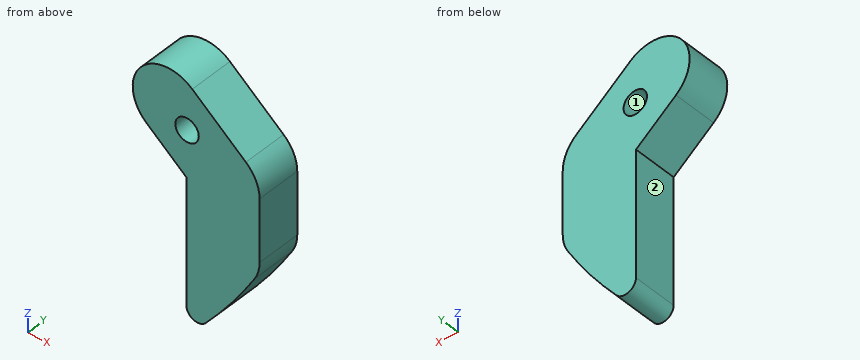
```python
from build123d import *

# Parameters (mm, degrees)
ESBO_O1_R                = 1.6
RESSALTO_EXTRUS_O1_DEPTH = 6


with BuildPart() as part:
    # Esboço1 → Ressalto-extrusão1 (new body)
    with BuildSketch(Plane.XZ.offset(12)):
        with BuildLine():
            Line((-5.554408486, -1.950425304), (-0.098401843, -6.33585476))
            Line((-0.098401843, -6.33585476), (-0.098401843, -23.434191187))
            ThreePointArc((-0.098401843, -23.434191187), (0.884517689, -24.84224935), (2.545101876, -24.404963685))
            ThreePointArc((2.545101876, -24.404963685), (6.090429059, -19.835978921), (9.220727662, -14.973243345))
            ThreePointArc((9.220727662, -14.973243345), (9.728380083, -13.758965882), (9.901598157, -12.454291119))
            Line((9.901598157, -12.454291119), (9.901598157, -3.939806958))
            ThreePointArc((9.901598157, -3.939806958), (9.410602928, -1.779048764), (8.034047768, -0.042659356))
            Line((8.034047768, -0.042659356), (0.710490736, 5.843869901))
            ThreePointArc((0.710490736, 5.843869901), (-6.319106477, 5.07917191), (-5.554408486, -1.950425304))
        make_face()
        with Locations(Location((0, 0, 0), (0, 0, 90))):
            Circle(ESBO_O1_R, mode=Mode.SUBTRACT)
    extrude(amount=-RESSALTO_EXTRUS_O1_DEPTH)


solid = part.part
```
CAD build for the part. Positions are in the model's coordinates, mm. Face numbers are marked on the shaded views. A direction names the side the tool comes from. Round coordinates to 2 decimals unless told otherwise and drop trailing zeros. Write each loop counter-clockwise with the first axis right and the second up, starting at its lowest first coordinate (ties: lowest second). Pieces come first, ordered by that corner, then holes.
Item 1: Band-saw the part on C-C on x = 4.75. Write the cut outline in (y, z).
Filled in:
outline: (-12, -21.66) - (-6, -21.66) - (-6, 2.6) - (-12, 2.6) - close
Item 2: Tool access for the marked faces 1 and 2: list every direction of +Z, -Z, +X, -X, +Y, -Y with a clear straight run to the whole face (end or side of a thin tool).
Filled in:
face 1: +Y, -Y
face 2: -Z, -X, +Y, -Y
Item 3: Band-saw the part on B-B on z = -9. Write the cut outline in (x, y), then the cut area to 3 significant figures.
Filled in:
outline: (-0.1, -12) - (9.9, -12) - (9.9, -6) - (-0.1, -6) - close
area: 60.0 mm2
Item 4: Drill centre lines: L1, parallel to X at y = -9.95, z = -9.5; L2, parallel to X at y = -9.6, z = 0; L3, parallel to Z at x = 6, y = -8.15. Where is each one in solid material? Low to high.
Filled in:
L1: x = -0.1 to 9.9
L2: x = -7.03 to -1.6, 1.6 to 7.98
L3: z = -19.96 to 1.59
Item 5: Drop flat-ended pins along their axis: pin 1 Ø1 at (y, z) = (-7, -1.5) entering from +X; pin 2 Ø3 at (y, z) = (-9, -15) entering from -X. Give the stop position or say it passes through.
Filled in:
pin 1: stops at x = 9.51
pin 2: stops at x = -0.1
